Work out the finished part from the listing and answer in its coordinate system (mm). A direction names the side the tool comes from. Round coordinates to 2 decimals unless told otherwise and drop trailing zeros. Loops run counter-clockwise (first coordinate to the right, second up) from the corner with the lowest first, then second, coordinate; pieces in that order, holes last.
```python
from build123d import *

# Parameters (mm, degrees)
SKETCH1_R           = 58
SKETCH1_R_2         = 1.7
BOSS_EXTRUDE1_DEPTH = 3
CUT_EXTRUDE1_DEPTH  = 83.079230016


with BuildPart() as part:
    # Sketch1 → Boss-Extrude1 (new body)
    with BuildSketch(Plane.XY):
        Circle(SKETCH1_R)
        with Locations((0, 53)):
            Circle(SKETCH1_R_2, mode=Mode.SUBTRACT)
        with Locations((45.899346401, -26.5)):
            Circle(SKETCH1_R_2, mode=Mode.SUBTRACT)
        with Locations((-45.899346401, -26.5)):
            Circle(SKETCH1_R_2, mode=Mode.SUBTRACT)
    extrude(amount=BOSS_EXTRUDE1_DEPTH)

    # Sketch2 → Cut-Extrude1 (cut, through all)
    with BuildSketch(Plane.XY.offset(3)):
        with BuildLine():
            Line((-3.5, 45), (3.5, 45))
            ThreePointArc((3.5, 45), (6.5, 42), (3.5, 39))
            Line((3.5, 39), (-3.5, 39))
            ThreePointArc((-3.5, 39), (-6.5, 42), (-3.5, 45))
        make_face()
    extrude(amount=-CUT_EXTRUDE1_DEPTH, mode=Mode.SUBTRACT)


solid = part.part
```
1. Consider probe 1 along Y at (x, z) = (3.5, 2.45); probe 2 along Y at (x, z) = (47, 0.3); probe 3 along X at (y, z) = (-31, 1.85). Determine where each line is inside the solid, lowest interval first.
Answer key:
probe 1: y = -57.89 to 39, 45 to 57.89
probe 2: y = -33.99 to -27.8, -25.2 to 33.99
probe 3: x = -49.02 to 49.02
2. Find section B-B (y = 42). Write down the section's boundary in (x, z), then the cut area to 3 significant figures.
Answer key:
outline: (-40, 0) - (-6.5, 0) - (-6.5, 3) - (-40, 3) - close; (6.5, 0) - (40, 0) - (40, 3) - (6.5, 3) - close
area: 201 mm2
3. Which of the six approach directions +Z, -Z, +X, -X, +Y, -Y give full straight-line access (tool end or side, diameter ignored) to faces 4 (the face through (-1, 1, 3)), 5 (the face through (0, 39, 2))?
Answer key:
face 4: +Z, +X, -X, +Y, -Y
face 5: +Z, -Z
4. Find section D-D (y = -26.5). Write down the section's boundary in (x, z).
Answer key:
outline: (-51.59, 0) - (-47.6, 0) - (-47.6, 3) - (-51.59, 3) - close; (-44.2, 0) - (44.2, 0) - (44.2, 3) - (-44.2, 3) - close; (47.6, 0) - (51.59, 0) - (51.59, 3) - (47.6, 3) - close
5. Find section C-C (z = 1.25). Write down the section's boundary in (x, y).
Answer key:
outline: circle Ø116 at (0, 0); hole circle Ø3.4 at (-45.9, -26.5); hole (-3.5, 39) - (3.5, 39) arc R3 ccw to (3.5, 45) - (-3.5, 45) arc R3 ccw to start; hole circle Ø3.4 at (0, 53); hole circle Ø3.4 at (45.9, -26.5)
6. Given pin 1 (1 mm diameter, centred on x = 45, z = 0.5, fed in from +Y); pin 2 (2.5 mm diameter, centred on x = 0, y = 53, fed in from -Z); pin 3 (1.5 mm diameter, centred on x = -1.5, z = 1.5, fed in from -Y), each flat-ended and moving along its own axis, determine where each tip first touches the part or whether it passes through.
Answer key:
pin 1: stops at y = 37.2
pin 2: passes through
pin 3: stops at y = -58
7. Find section A-A (x = 0). Write down the section's boundary in (y, z), then the cut area to 3 significant figures.
Answer key:
outline: (-58, 0) - (39, 0) - (39, 3) - (-58, 3) - close; (45, 0) - (51.3, 0) - (51.3, 3) - (45, 3) - close; (54.7, 0) - (58, 0) - (58, 3) - (54.7, 3) - close
area: 320 mm2
8. Determine the mould class of faces 1 (the face through (-6.5, 41.9, 1.5)), 2 (the face through (-1, 1, 0)), 3 (the face through (26.76, -51.46, 1.48)) for opening direction Y: +Y half, -Y half, draft (parallel to the pull), parting line (faces both ways), or undercut.
Answer key:
face 1: undercut
face 2: draft
face 3: parting line
